from build123d import *

# Parameters (mm, degrees)
S01_INNER_RACE_CONTACT_LIPS_R         = 21
S01_INNER_RACE_CONTACT_LIPS_R_2       = 20.12
F_01_INNER_RACE_CONTACT_LIPS_DEPTH    = 6
F_02_START                            = 1
S02_STIFFENED_MIDDLE_OF_SPACER_R      = 21.9
S02_STIFFENED_MIDDLE_OF_SPACER_R_2    = 20.12
F_02_STIFFENED_MIDDLE_OF_SPACER_DEPTH = 4


with BuildPart() as part:
    # S01 - Inner race contact lips → 01 - Inner race contact lips (new body)
    with BuildSketch(Plane.XY):
        Circle(S01_INNER_RACE_CONTACT_LIPS_R)
        Circle(S01_INNER_RACE_CONTACT_LIPS_R_2, mode=Mode.SUBTRACT)
    extrude(amount=F_01_INNER_RACE_CONTACT_LIPS_DEPTH)

    # S02 - Stiffened middle of spacer → 02 - Stiffened middle of spacer (add)
    with BuildSketch(Plane.XY.offset(F_02_START)):
        Circle(S02_STIFFENED_MIDDLE_OF_SPACER_R)
        Circle(S02_STIFFENED_MIDDLE_OF_SPACER_R_2, mode=Mode.SUBTRACT)
    extrude(amount=F_02_STIFFENED_MIDDLE_OF_SPACER_DEPTH)


solid = part.part
The listing builds one solid part. Answer for the finished solid, in the listing's coordinates (mm). A direction names the side the tool comes from. Give positions to 0.01 mm unless a question says otherwise; leave off trailing zeros. Write each loop counter-clockwise with the first axis right and the second up, starting at its lowest first coordinate (ties: lowest second). Pieces come first, ordered by that corner, then holes.
Item 1: Section C-C, the plane z = 4.3 is taken. Write down the section's boundary in (x, y).
Item 2: Determine the mould class of faces 3 (the cylindrical face through (20.03, 6.31, 0.49)), 4 (the cylindrical face through (-2.62, 19.95, 2.96)) for opening direction Y: released by +Y, released by -Y, zero draft, split by the parting line, or undercut.
Item 3: Section A-A, the plane x = 0 is taken. Write down the section's boundary in (y, z).
Item 4: Flat-ended cylindrical pins translate along their axes: P1, Ø2, axis at y = 14.5, z = 1, coming from the -X side; P2, Ø1.5, axis at y = -9.5, z = 2.5, coming from the +X side; P3, Ø3, axis at y = -3.5, z = 4.5, coming from the -X side. Find the tip coordinate at first contact, or state that the pin passes through.
Item 5: Which of the six approach directions +Z, -Z, +X, -X, +Y, -Y give full straight-line access (tool end or side, diameter ignored) to faces 1 (the cylindrical face through (-17.4, -13.3, 3)), 2 (the cylindrical face through (20.03, 6.31, 5.49))?
Item 6: Find the intervals of material crossed by line 1 along X through (y, z) = (-0.5, 3.4); line 2 along Z through (x, y) = (16.5, -14); line 3 along Y through (x, z) = (0, 4.15), in increasing order.
Completed:
1. outline: circle Ø43.8 at (0, 0); hole circle Ø40.24 at (0, 0)
2. face 3: split by the parting line
2. face 4: undercut
3. outline: (-21.9, 1) - (-21, 1) - (-21, 0) - (-20.12, 0) - (-20.12, 6) - (-21, 6) - (-21, 5) - (-21.9, 5) - close; (20.12, 0) - (21, 0) - (21, 1) - (21.9, 1) - (21.9, 5) - (21, 5) - (21, 6) - (20.12, 6) - close
4. P1: stops at x = -17.24
4. P2: stops at x = 20.08
4. P3: stops at x = -21.81
5. face 1: +Z, -Z
5. face 2: +Z
6. line 1: x = -21.89 to -20.11, 20.11 to 21.89
6. line 2: z = 1 to 5
6. line 3: y = -21.9 to -20.12, 20.12 to 21.9
